```python
from build123d import *

# Parameters (mm, degrees)
SKETCH_1_R          = 22
EXTRUDE_1_DEPTH     = 2
SKETCH_2_R          = 12.45
SKETCH_2_R_2        = 10
EXTRUDE_2_DEPTH     = 2
SKETCH_3_R          = 2.9
CUT_EXTRUDE_1_DEPTH = 11
EXTRUDE_3_DEPTH     = 3
SKETCH_5_R          = 0.6
CUT_EXTRUDE_2_DEPTH = 16
SKETCH_6_R          = 14.5
SKETCH_6_R_2        = 4
EXTRUDE_4_DEPTH     = 0.4


with BuildPart() as part:
    # 草图1 → 凸台-拉伸1 (new body)
    with BuildSketch(Plane.XY):
        Circle(SKETCH_1_R)
    extrude(amount=EXTRUDE_1_DEPTH)

    # 草图2 → 凸台-拉伸2 (add)
    with BuildSketch(Plane.XY.offset(2)):
        Circle(SKETCH_2_R)
        Circle(SKETCH_2_R_2, mode=Mode.SUBTRACT)
    extrude(amount=EXTRUDE_2_DEPTH)

    # 草图3 → 切除-拉伸1 (cut)
    with BuildSketch(Plane.XY.offset(2)):
        Circle(SKETCH_3_R)
    extrude(amount=-CUT_EXTRUDE_1_DEPTH, mode=Mode.SUBTRACT)

    # 草图4 → 凸台-拉伸3 (add)
    with BuildSketch(Plane(origin=(0, 0, 0), x_dir=(-1, 0, 0), z_dir=(0, 0, -1))):
        with BuildLine():
            ThreePointArc((1.369754339, -21.957317073), (0, -18.5), (-1.369754339, -21.957317073))
            ThreePointArc((-1.369754339, -21.957317073), (0, -22), (1.369754339, -21.957317073))
        make_face()
        with BuildLine():
            ThreePointArc((-19.700471554, 9.792416482), (-16.02146997, 9.25), (-18.330717215, 12.164900591))
            ThreePointArc((-18.330717215, 12.164900591), (-19.052558883, 11), (-19.700471554, 9.792416482))
        make_face()
        with BuildLine():
            ThreePointArc((18.330717215, 12.164900591), (16.02146997, 9.25), (19.700471554, 9.792416482))
            ThreePointArc((19.700471554, 9.792416482), (19.052558883, 11), (18.330717215, 12.164900591))
        make_face()
    extrude(amount=EXTRUDE_3_DEPTH)

    # 草图5 → 切除-拉伸2 (cut)
    with BuildSketch(Plane(origin=(0, 0, -3), x_dir=(-1, 0, 0), z_dir=(0, 0, -1))):
        with Locations((0, -20.5)):
            Circle(SKETCH_5_R)
        with Locations((-17.753520778, 10.25)):
            Circle(SKETCH_5_R)
        with Locations((17.753520778, 10.25)):
            Circle(SKETCH_5_R)
    extrude(amount=-CUT_EXTRUDE_2_DEPTH, mode=Mode.SUBTRACT)

    # 草图6 → 凸台-拉伸4 (add)
    with BuildSketch(Plane.XY.offset(2)):
        Circle(SKETCH_6_R)
        Circle(SKETCH_6_R_2, mode=Mode.SUBTRACT)
    extrude(amount=EXTRUDE_4_DEPTH)


solid = part.part
```
CAD build for the part. Positions are in the model's coordinates, mm. A direction names the side the tool comes from. Round coordinates to 2 decimals unless told otherwise and drop trailing zeros. Write each loop counter-clockwise with the first axis right and the second up, starting at its lowest first coordinate (ties: lowest second). Pieces come first, ordered by that corner, then holes. Notation, with made-up numbers: (-36, 15.5) - (-11, 15.5) arc R3 ccw to (-11, 19.5) - close; hole circle Ø7 at (-24.75, 7.25). An arc over 180 degrees is marked (long way). Return JSON: item names as keys, results as strings. Group by question number.
Item 1: Band-saw the part on B-B on y = 0. List the corners of the cut face in (x, z), plus the area to 3 significant figures.
Item 2: Flat gauge pins, fed straight in: pin 1 Ø7 at (x, y) = (0, 0) entering from -Z; pin 2 Ø1.5 at (x, z) = (8, -0.5) entering from +Y; pin 3 Ø6.5 at (x, y) = (0, 0) entering from +Z; pin 4 Ø1 at (x, y) = (0, -20.5) entering from +Z. Where does each tip first touch, or does it go through?
Item 3: Band-saw the part on D-D on y = 5.5. List the corners of the cut face in (x, z).
Item 4: 3-axis set-ups, long thin cutter, end or side, ignore diameter. For faces 4 (the face through (-17, 10, -3)), 5 (the face through (6.691, -12.864, 2.197)), 6 (the face through (-15.99, 9.31, -1.48)): which of +Z, -Z, +X, -X, +Y, -Y reach the whole face in a straight line?
Item 5: Mould opens along Y. For faces 1 (the face through (16.056, 9.193, -1.479)), 2 (the face through (-0.867, -3.905, 2.197)), 3 (the face through (0, -5, 0)) say: +Y half, -Y half, draft (parallel to the pull), parting line (faces both ways), or undercut.
Item 6: Band-saw the part on A-A on x = 0. State how many separate pieces and enclosed holes the cut face has, plus the area to 3 significant figures.
Item 7: Band-saw the part on C-C on x = 7.5. List the corners of the cut face in (y, z).
Item 8: Probe probe 1 along Y at (x, z) = (0, 3.2); probe 2 along Z at (x, y) = (-11.5, 3). List the from-to ranges inside material, lowest first.
Resolved:
{
 "1": {"outline": "(-22, 0) - (-2.9, 0) - (-2.9, 2) - (-4, 2) - (-4, 2.4) - (-10, 2.4) - (-10, 4) - (-12.45, 4) - (-12.45, 2.4) - (-14.5, 2.4) - (-14.5, 2) - (-22, 2) - close; (2.9, 0) - (22, 0) - (22, 2) - (14.5, 2) - (14.5, 2.4) - (12.45, 2.4) - (12.45, 4) - (10, 4) - (10, 2.4) - (4, 2.4) - (4, 2) - (2.9, 2) - close", "area": "92.6 mm²"},
 "2": {"pin 1": "stops at z = 0", "pin 2": "stops at y = 20.7", "pin 3": "stops at z = 2", "pin 4": "passes through"},
 "3": {"outline": "(-21.3, 0) - (21.3, 0) - (21.3, 2) - (13.42, 2) - (13.42, 2.4) - (11.17, 2.4) - (11.17, 4) - (8.35, 4) - (8.35, 2.4) - (-8.35, 2.4) - (-8.35, 4) - (-11.17, 4) - (-11.17, 2.4) - (-13.42, 2.4) - (-13.42, 2) - (-21.3, 2) - close"},
 "4": {"face 4": "-Z, +X, -X, +Y, -Y", "face 5": "+Z", "face 6": "-Z"},
 "5": {"face 1": "parting line", "face 2": "undercut", "face 3": "draft"},
 "6": {"separate pieces": "3", "enclosed holes": "0", "area": "97.1 mm²"},
 "7": {"outline": "(-20.68, 0) - (20.68, 0) - (20.68, 2) - (12.41, 2) - (12.41, 2.4) - (9.94, 2.4) - (9.94, 4) - (6.61, 4) - (6.61, 2.4) - (-6.61, 2.4) - (-6.61, 4) - (-9.94, 4) - (-9.94, 2.4) - (-12.41, 2.4) - (-12.41, 2) - (-20.68, 2) - close"},
 "8": {"probe 1": "y = -12.45 to -10, 10 to 12.45", "probe 2": "z = 0 to 4"}
}
